Can you work these out from the model? Positions are in its coordinate system, mm. A direction names the side the tool comes from. Round coordinates to 2 decimals unless told otherwise and drop trailing zeros. Loops run counter-clockwise (first coordinate to the right, second up) from the corner with the lowest first, then second, coordinate; pieces in that order, holes last.
from build123d import *

# Parameters (mm, degrees)
BOSS_EXTRUDE1_DEPTH = 40
FILLET1_R           = 3
SHELL1_T            = -1
SKETCH2_W           = 65
SKETCH2_H           = 15
CUT_EXTRUDE1_DEPTH  = 53.201532545
VENT1_START         = -12.137690598
VENT1_OUTLINE_W     = 4
VENT1_OUTLINE_H     = 10
VENT1_OUTLINE_W_2   = 3
VENT1_DEPTH         = 1
VENT1_2_OUTLINE_W   = 2
VENT1_2_OUTLINE_H   = 10
VENT1_2_DEPTH       = 0.5


# Read off the part's stored shape, not the designer's step: Vent1
with BuildPart() as part:
    # Sketch1 → Boss-Extrude1 (new, symmetric)
    with BuildSketch(Plane.XY):
        with BuildLine():
            Line((-5.751201461, 27.808889777), (-12.137690598, 5))
            Line((-12.137690598, 5), (-12.137690598, -30))
            Line((-12.137690598, -30), (2.862309402, -30))
            Line((2.862309402, -30), (2.862309402, 30))
            Line((2.862309402, 30), (-2.862309402, 30))
            ThreePointArc((-2.862309402, 30), (-4.675225653, 29.390258284), (-5.751201461, 27.808889777))
        make_face()
    extrude(amount=BOSS_EXTRUDE1_DEPTH, both=True)

    # Fillet1
    fillet1_edges = [part.edges().sort_by_distance(p)[0] for p in [
        (-12.137690598, 5, 0),
        (-4.675225653, 29.390258284, 40),
        (-8.94444603, 16.404444888, 40),
        (-12.137690598, -12.5, 40),
        (-12.137690598, -12.5, -40),
        (-8.94444603, 16.404444888, -40),
        (-4.675225653, 29.390258284, -40),
        (0, 30, -40),
        (0, 30, 40),
    ]]
    fillet(fillet1_edges, radius=FILLET1_R)

    # Shell1
    shell1_openings = [part.faces().sort_by_distance(p)[0] for p in [
        (2.862309402, -0.023622446, 0),
    ]]
    offset(amount=SHELL1_T, openings=shell1_openings, kind=Kind.INTERSECTION)

    # Sketch2 → Cut-Extrude1 (cut, through all)
    with BuildSketch(Plane.ZY.offset(12.137690598)):
        with Locations((0, 15.5)):
            Rectangle(SKETCH2_W, SKETCH2_H)
    extrude(amount=-CUT_EXTRUDE1_DEPTH, mode=Mode.SUBTRACT)

    # Vent1 outline → Vent1 (cut)
    with BuildSketch(Plane.YZ.offset(VENT1_START)):
        with BuildLine():
            add(Edge.make_bspline(
                [(-20, 17.5), (-20, 18.484636289), (-19.807852804, 19.45090322), (-19.615866008, 20.416363534), (-19.238795325, 21.326834324), (-18.862145538, 22.236288823), (-18.314696123, 23.05570233), (-17.767857785, 23.874201188), (-17.071067812, 24.571067812), (-16.567779985, 25.074411003), (-16, 25.500081295)],
                knots=[0, 0, 0, 0.0625, 0.0625, 0.125, 0.125, 0.1875, 0.1875, 0.25, 0.25, 0.295193876, 0.295193876, 0.295193876], degree=2))
            Line((-20, 17.5), (-20, 13))
            Line((-20, 13), (-16, 13))
            Line((-16, 13), (-16, 25.500081295))
        make_face()
        with BuildLine():
            add(Edge.make_bspline(
                [(-14, 26.665158313), (-13.9138372, 26.702751948), (-13.826834324, 26.738795325), (-12.917421262, 27.11554515), (-11.95090322, 27.307852804), (-11.477855415, 27.40197491), (-11, 27.449991893)],
                knots=[0.369027345, 0.369027345, 0.369027345, 0.375, 0.375, 0.4375, 0.4375, 0.468123874, 0.468123874, 0.468123874], degree=2))
            Line((-14, 26.665158313), (-14, 13))
            Line((-14, 13), (-11, 13))
            Line((-11, 13), (-11, 27.449991893))
        make_face()
        with BuildLine():
            add(Edge.make_bspline(
                [(-9, 27.449990782), (-8.522411136, 27.401973821), (-8.04909678, 27.307852804), (-7.083636466, 27.115866008), (-6.173165676, 26.738795325), (-6.086170897, 26.702766513), (-6, 26.665174873)],
                knots=[0.531893743, 0.531893743, 0.531893743, 0.5625, 0.5625, 0.625, 0.625, 0.6309785, 0.6309785, 0.6309785], degree=2))
            Line((-9, 27.449990782), (-9, 13))
            Line((-9, 13), (-6, 13))
            Line((-6, 13), (-6, 26.665174873))
        make_face()
        with BuildLine():
            add(Edge.make_bspline(
                [(-4, 25.500105578), (-3.432685944, 25.074766157), (-2.928932188, 24.571067812), (-2.232843424, 23.875055613), (-1.685303877, 23.05570233), (-1.138375507, 22.23726363), (-0.761204675, 21.326834324), (-0.38445485, 20.417421262), (-0.192147196, 19.45090322), (0, 18.485191624), (0, 17.5)],
                knots=[0.704819748, 0.704819748, 0.704819748, 0.75, 0.75, 0.8125, 0.8125, 0.875, 0.875, 0.9375, 0.9375, 1, 1, 1], degree=2))
            Line((-4, 25.500105578), (-4, 13))
            Line((-4, 13), (0, 13))
            Line((0, 13), (0, 17.5))
        make_face()
        with BuildLine():
            add(Edge.make_bspline(
                [(0, -17.5), (0, -18.484636289), (-0.192147196, -19.45090322), (-0.384133992, -20.416363534), (-0.761204675, -21.326834324), (-1.137854462, -22.236288823), (-1.685303877, -23.05570233), (-2.232142215, -23.874201188), (-2.928932188, -24.571067812), (-3.432220015, -25.074411003), (-4, -25.500081295)],
                knots=[0, 0, 0, 0.0625, 0.0625, 0.125, 0.125, 0.1875, 0.1875, 0.25, 0.25, 0.295193876, 0.295193876, 0.295193876], degree=2))
            Line((0, -17.5), (0, -13))
            Line((0, -13), (-4, -13))
            Line((-4, -13), (-4, -25.500081295))
        make_face()
        with BuildLine():
            add(Edge.make_bspline(
                [(-6, -26.665158313), (-6.086162801, -26.702751948), (-6.173165676, -26.738795325), (-7.082578738, -27.11554515), (-8.04909678, -27.307852804), (-8.522144585, -27.40197491), (-9, -27.449991893)],
                knots=[0.369027345, 0.369027345, 0.369027345, 0.375, 0.375, 0.4375, 0.4375, 0.468123874, 0.468123874, 0.468123874], degree=2))
            Line((-6, -26.665158313), (-6, -13))
            Line((-6, -13), (-9, -13))
            Line((-9, -13), (-9, -27.449991893))
        make_face()
        with BuildLine():
            add(Edge.make_bspline(
                [(-11, -27.449990782), (-11.477588864, -27.401973821), (-11.95090322, -27.307852804), (-12.916363534, -27.115866008), (-13.826834324, -26.738795325), (-13.913829103, -26.702766513), (-14, -26.665174873)],
                knots=[0.531893743, 0.531893743, 0.531893743, 0.5625, 0.5625, 0.625, 0.625, 0.6309785, 0.6309785, 0.6309785], degree=2))
            Line((-11, -27.449990782), (-11, -13))
            Line((-11, -13), (-14, -13))
            Line((-14, -13), (-14, -26.665174873))
        make_face()
        with BuildLine():
            add(Edge.make_bspline(
                [(-16, -25.500105578), (-16.567314056, -25.074766157), (-17.071067812, -24.571067812), (-17.767156576, -23.875055613), (-18.314696123, -23.05570233), (-18.861624493, -22.23726363), (-19.238795325, -21.326834324), (-19.61554515, -20.417421262), (-19.807852804, -19.45090322), (-20, -18.485191624), (-20, -17.5)],
                knots=[0.704819748, 0.704819748, 0.704819748, 0.75, 0.75, 0.8125, 0.8125, 0.875, 0.875, 0.9375, 0.9375, 1, 1, 1], degree=2))
            Line((-16, -25.500105578), (-16, -13))
            Line((-16, -13), (-20, -13))
            Line((-20, -13), (-20, -17.5))
        make_face()
        with Locations((-2, -6)):
            Rectangle(VENT1_OUTLINE_W, VENT1_OUTLINE_H)
        with Locations((-7.5, -6)):
            Rectangle(VENT1_OUTLINE_W_2, VENT1_OUTLINE_H)
        with Locations((-12.5, -6)):
            Rectangle(VENT1_OUTLINE_W_2, VENT1_OUTLINE_H)
        with Locations((-18, -6)):
            Rectangle(VENT1_OUTLINE_W, VENT1_OUTLINE_H)
        with Locations((-2, 6)):
            Rectangle(VENT1_OUTLINE_W, VENT1_OUTLINE_H)
        with Locations((-7.5, 6)):
            Rectangle(VENT1_OUTLINE_W_2, VENT1_OUTLINE_H)
        with Locations((-12.5, 6)):
            Rectangle(VENT1_OUTLINE_W_2, VENT1_OUTLINE_H)
        with Locations((-18, 6)):
            Rectangle(VENT1_OUTLINE_W, VENT1_OUTLINE_H)
    extrude(amount=VENT1_DEPTH, mode=Mode.SUBTRACT)

    # Vent1 2 outline → Vent1 2 (cut)
    with BuildSketch(Plane.YZ.offset(VENT1_START)):
        with BuildLine():
            add(Edge.make_bspline(
                [(-16, 25.500081295), (-15.782579599, 25.663083528), (-15.55570233, 25.814696123), (-14.815475656, 26.309358665), (-14, 26.665158313)],
                knots=[0.295193876, 0.295193876, 0.295193876, 0.3125, 0.3125, 0.369027345, 0.369027345, 0.369027345], degree=2))
            Line((-16, 25.500081295), (-16, 13))
            Line((-16, 13), (-14, 13))
            Line((-14, 13), (-14, 26.665158313))
        make_face()
        with BuildLine():
            add(Edge.make_bspline(
                [(-11, 27.449991893), (-10.502604415, 27.499972357), (-10, 27.5), (-9.497679153, 27.500027628), (-9, 27.449990782)],
                knots=[0.468123874, 0.468123874, 0.468123874, 0.5, 0.5, 0.531893743, 0.531893743, 0.531893743], degree=2))
            Line((-11, 27.449991893), (-11, 13))
            Line((-11, 13), (-9, 13))
            Line((-9, 13), (-9, 27.449990782))
        make_face()
        with BuildLine():
            add(Edge.make_bspline(
                [(-6, 26.665174873), (-5.18532936, 26.309778717), (-4.44429767, 25.814696123), (-4.217478567, 25.663158488), (-4, 25.500105578)],
                knots=[0.6309785, 0.6309785, 0.6309785, 0.6875, 0.6875, 0.704819748, 0.704819748, 0.704819748], degree=2))
            Line((-6, 26.665174873), (-6, 13))
            Line((-6, 13), (-4, 13))
            Line((-4, 13), (-4, 25.500105578))
        make_face()
        with BuildLine():
            add(Edge.make_bspline(
                [(-4, -25.500081295), (-4.217420401, -25.663083528), (-4.44429767, -25.814696123), (-5.184524344, -26.309358665), (-6, -26.665158313)],
                knots=[0.295193876, 0.295193876, 0.295193876, 0.3125, 0.3125, 0.369027345, 0.369027345, 0.369027345], degree=2))
            Line((-4, -25.500081295), (-4, -13))
            Line((-4, -13), (-6, -13))
            Line((-6, -13), (-6, -26.665158313))
        make_face()
        with BuildLine():
            add(Edge.make_bspline(
                [(-9, -27.449991893), (-9.497395585, -27.499972357), (-10, -27.5), (-10.502320847, -27.500027628), (-11, -27.449990782)],
                knots=[0.468123874, 0.468123874, 0.468123874, 0.5, 0.5, 0.531893743, 0.531893743, 0.531893743], degree=2))
            Line((-9, -27.449991893), (-9, -13))
            Line((-9, -13), (-11, -13))
            Line((-11, -13), (-11, -27.449990782))
        make_face()
        with BuildLine():
            add(Edge.make_bspline(
                [(-14, -26.665174873), (-14.81467064, -26.309778717), (-15.55570233, -25.814696123), (-15.782521433, -25.663158488), (-16, -25.500105578)],
                knots=[0.6309785, 0.6309785, 0.6309785, 0.6875, 0.6875, 0.704819748, 0.704819748, 0.704819748], degree=2))
            Line((-14, -26.665174873), (-14, -13))
            Line((-14, -13), (-16, -13))
            Line((-16, -13), (-16, -25.500105578))
        make_face()
        with Locations((-5, -6)):
            Rectangle(VENT1_2_OUTLINE_W, VENT1_2_OUTLINE_H)
        with Locations((-10, -6)):
            Rectangle(VENT1_2_OUTLINE_W, VENT1_2_OUTLINE_H)
        with Locations((-15, -6)):
            Rectangle(VENT1_2_OUTLINE_W, VENT1_2_OUTLINE_H)
        with Locations((-5, 6)):
            Rectangle(VENT1_2_OUTLINE_W, VENT1_2_OUTLINE_H)
        with Locations((-10, 6)):
            Rectangle(VENT1_2_OUTLINE_W, VENT1_2_OUTLINE_H)
        with Locations((-15, 6)):
            Rectangle(VENT1_2_OUTLINE_W, VENT1_2_OUTLINE_H)
    extrude(amount=VENT1_2_DEPTH, mode=Mode.SUBTRACT)


solid = part.part
(1) Will these pins go through, and if not, where does the flat tip stop? P1, Ø1.1, axis at x = -11, z = -12.5, coming from the +Y side; P2, Ø2, axis at y = -15.5, z = 4, coming from the -X side; P3, Ø4, axis at y = 3, z = -25.5, coming from the +X side.
Worked answers:
P1: stops at y = 8
P2: stops at x = -11.64
P3: stops at x = -11.09
(2) If I drill on line 1 (Y direction, x = -1.75, z = 2); line 2 (Z direction, x = -5.75, y = -8); line 3 (X direction, y = -4.5, z = 3), over which ranges is the centre line in solid material (lowest first)?
Worked answers:
line 1: y = -30 to -29, 29 to 30
line 2: z = -40 to -39, 39 to 40
line 3: x = -11.64 to -11.14
(3) If we section it at A-A, the plane z = -2.5: State how many separate pieces and enclosed holes the cut face has, then the cut area to 3 significant figures.
Worked answers:
separate pieces: 6
enclosed holes: 0
area: 48.9 mm2
(4) If we mould it in two halves opening along Z, with no side actions, what happens to faces 4 (the cylindrical face through (-10.567, -12.441, -38.399)), 5 (the cylindrical face through (-8.109, 16.215, -39.098))? For each: released by +Z, released by -Z, zero draft, split by the parting line, or undercut.
Worked answers:
face 4: undercut
face 5: released by -Z
(5) If we section it at B-B, the plane y = 1.5: List the corners of the cut face in (x, z) for me.
Worked answers:
outline: (-12.14, -37) arc R3 ccw to (-9.14, -40) - (2.86, -40) - (2.86, -39) - (-9.14, -39) arc R2 cw to (-11.14, -37) - (-11.14, 37) arc R2 cw to (-9.14, 39) - (2.86, 39) - (2.86, 40) - (-9.14, 40) arc R3 ccw to (-12.14, 37) - close
(6) For faces 1 (the cylindrical face through (-0.04, 29.14, -39.1)), 2 (the flat face through (-4, -29, 1)), 3 (the flat face through (-11.638, -15, -6)), which set-ups out of +Z, -Z, +X, -X, +Y, -Y let a thin tool reach every point of the face, with its end or its side?
Worked answers:
face 1: -Z, +X, -X, +Y
face 2: +X
face 3: -X
